from build123d import *

# Parameters (mm, degrees)
SPROCKET_R                   = 45
ESTRUSIONE_ESTRUSIONE2_DEPTH = 3
SCHIZZO4_R                   = 10
ESTRUSIONE_ESTRUSIONE4_DEPTH = 12
SCHIZZO5_R                   = 29
SCHIZZO5_R_2                 = 28
ESTRUSIONE_ESTRUSIONE5_DEPTH = 12
SCHIZZO6_R                   = 3.175
TAGLIO_ESTRUSIONE1_DEPTH     = 15
RACCORDO1_R                  = 6.5
SCHIZZO7_R                   = 6.5
SCHIZZO7_R_2                 = 2.5
TAGLIO_ESTRUSIONE2_DEPTH     = 4
SCALE1_SCALE                 = 0.888888889


with BuildPart() as part:
    # Sprocket → Estrusione-Estrusione2 (new body)
    with BuildSketch(Plane(origin=(0, 0, 0), x_dir=(0, 0, -1), z_dir=(1, 0, 0))):
        Circle(SPROCKET_R)
    extrude(amount=ESTRUSIONE_ESTRUSIONE2_DEPTH)

    # Schizzo4 → Estrusione-Estrusione4 (add)
    with BuildSketch(Plane(origin=(3, 0, 0), x_dir=(0, 0, -1), z_dir=(1, 0, 0))):
        Circle(SCHIZZO4_R)
    extrude(amount=ESTRUSIONE_ESTRUSIONE4_DEPTH)

    # Schizzo5 → Estrusione-Estrusione5 (add)
    with BuildSketch(Plane(origin=(3, 0, 0), x_dir=(0, 0, -1), z_dir=(1, 0, 0))):
        Circle(SCHIZZO5_R)
        Circle(SCHIZZO5_R_2, mode=Mode.SUBTRACT)
    extrude(amount=ESTRUSIONE_ESTRUSIONE5_DEPTH)

    # Schizzo6 → Taglio-Estrusione1 (cut)
    with BuildSketch(Plane(origin=(15, 0, 0), x_dir=(0, 0, -1), z_dir=(1, 0, 0))):
        Circle(SCHIZZO6_R)
    extrude(amount=-TAGLIO_ESTRUSIONE1_DEPTH, mode=Mode.SUBTRACT)

    # Raccordo1
    raccordo1_edges = [part.edges().sort_by_distance(p)[0] for p in [
        (3, 0, 10),
        (3, 0, 28),
    ]]
    fillet(raccordo1_edges, radius=RACCORDO1_R)

    # Schizzo7 → Taglio-Estrusione2 (cut, through all)
    with BuildSketch(Plane(origin=(3, 0, 0), x_dir=(0, 0, -1), z_dir=(1, 0, 0))):
        with Locations((0, 36.5)):
            Circle(SCHIZZO7_R)
        with Locations((36.5, 0)):
            Circle(SCHIZZO7_R)
        with Locations((0, -36.5)):
            Circle(SCHIZZO7_R)
        with Locations((-36.5, 0)):
            Circle(SCHIZZO7_R)
        with Locations((0, 19)):
            Circle(SCHIZZO7_R_2)
        with Locations((19, 0)):
            Circle(SCHIZZO7_R_2)
        with Locations((0, -19)):
            Circle(SCHIZZO7_R_2)
        with Locations((-19, 0)):
            Circle(SCHIZZO7_R_2)
    extrude(amount=-TAGLIO_ESTRUSIONE2_DEPTH, mode=Mode.SUBTRACT)


with BuildPart() as part_1:
    # Scale1: scaled about (3.427617089, 0, 0)
    add(part.part.scale(SCALE1_SCALE).moved(Location((0.380846343, 0, 0))))


solid = part_1.part
Input: part model. Units: mm. Frame: model coordinates. A direction names the side the tool comes from. Coordinates: 2 decimals unless noted, no trailing zeros. Loops run counter-clockwise (first coordinate to the right, second up) from the corner with the lowest first, then second, coordinate; pieces in that order, holes last. Notation, with made-up numbers: (-15, 16.5) - (44, 16.5) arc R16 ccw to (44, 30.5) - close; hole circle Ø6 at (31.25, 9). An arc over 180 degrees is marked (long way). Answer in a Markdown table with one row per item. Add a question column.
Item 1: Line query: line 1 along Y through (x, z) = (0.95, 0); line 2 along Y through (x, z) = (11, 0); line 3 along Y through (x, z) = (5.5, -2). Output: solid intervals per line, ascending. Write a range as [from, to].
Item 2: Contact query for flat-ended pins moving along their axis: P1, Ø4, axis at x = 9, z = -14.5, coming from the -Y side; P2, Ø6, axis at y = 16.89, z = 0, coming from the +X side; P3, Ø1.5, axis at x = 4, y = -14.5, coming from the +Z side. Output: stop coordinate, or through.
Item 3: Section query B-B on x = 6.25. Return the cut outline in (y, z).
Item 4: Mould query, pull axis Z, two halves, no side actions, for faces 3 (the cylindrical face through (1.7, -15.32, -36.95)), 4 (the flat face through (13.714, 21.1, 13.5)), 5 (the cylindrical face through (7.14, 0.85, -2.69)). Classes: released by +Z, released by -Z, zero draft, split by the parting line, or undercut.
Item 5: Access query for faces 1 (the cylindrical face through (11.236, -5.409, 7.054)), 2 (the cylindrical face through (1.73, -19.06, 0.48)). Directions: +Z, -Z, +X, -X, +Y, -Y. A direction counts if a zero-diameter tool reaches every point of the face in a straight line with its end or side. Return the directions, or none.
Item 6: Section query A-A on z = -29. Return the cut outline in (x, y), then the cut area to 3 significant figures.
Recorded:
| question | item | result |
|---|---|---|
| 1 | line 1 | [-40, -38.22], [-26.67, -19.11], [-14.67, -2.82], [2.82, 14.67], [19.11, 26.67], [38.22, 40] |
| 1 | line 2 | [-25.78, -24.89], [-8.89, -2.82], [2.82, 8.89], [24.89, 25.78] |
| 1 | line 3 | [-25.7, -23.75], [-9.74, -1.99], [1.99, 9.74], [23.75, 25.7] |
| 2 | P1 | y = -22.54 |
| 2 | P2 | x = 3.1 |
| 2 | P3 | z = 21.8 |
| 3 | outline | circle Ø51.56 at (0, 0); circle Ø18.99 at (0, 0); hole circle Ø48.57 at (0, 0); hole circle Ø5.64 at (0, 0) |
| 4 | face 3 | split by the parting line |
| 4 | face 4 | zero draft |
| 4 | face 5 | undercut |
| 5 | face 1 | +X |
| 5 | face 2 | +X, -X |
| 6 | outline | (0.38, -27.55) - (3.05, -27.55) - (3.05, -4.64) - (0.38, -4.64) - close; (0.38, 4.64) - (3.05, 4.64) - (3.05, 27.55) - (0.38, 27.55) - close |
| 6 | area | 122 mm^2 |
